```python
from build123d import *

# Parameters (mm, degrees)
ESQUISSE2_R             = 45
ESQUISSE2_R_2           = 1.55
BOSS_EXTRU_1_DEPTH      = 6.5
ENL_V_START             = -1.5
ESQUISSE3_R             = 45
ESQUISSE3_R_2           = 6
ENL_V_MAT_EXTRU_1_DEPTH = 1.5
CONG_1_R                = 0.1
ESQUISSE5_R             = 4
ENL_V_MAT_EXTRU_3_DEPTH = 5.5
SKETCH1_R               = 2.25
CUT_EXTRUDE1_DEPTH      = 64.835726815
SKETCH2_R               = 1.05
CUT_EXTRUDE2_DEPTH      = 64.970696557
CIRPATTERN1_COUNT       = 8
SKETCH6_R               = 6.9
CUT_EXTRUDE3_DEPTH      = 10
SKETCH7_R               = 5
CUT_EXTRUDE4_DEPTH      = 2.4


with BuildPart() as part:
    # Esquisse2 → Boss.-Extru.1 (new body)
    with BuildSketch(Plane(origin=(0, 0, 0), x_dir=(1, 0, 0), z_dir=(0, 1, 0))):
        with Locations(Location((0, 0, 0), (0, 0, 90))):
            Circle(ESQUISSE2_R)
        with Locations(Location((0, 0, 0), (0, 0, 90))):
            Circle(ESQUISSE2_R_2, mode=Mode.SUBTRACT)
    extrude(amount=BOSS_EXTRU_1_DEPTH)

    # Esquisse3 → Enlèv. mat.-Extru.1 (cut)
    with BuildSketch(Plane(origin=(0, 6.5, 0), x_dir=(1, 0, 0), z_dir=(0, 1, 0)).offset(ENL_V_START)):
        with Locations(Location((0, 0, 0), (0, 0, 90))):
            Circle(ESQUISSE3_R)
        with Locations(Location((0, 0, 0), (0, 0, 270))):
            Circle(ESQUISSE3_R_2, mode=Mode.SUBTRACT)
    extrude(amount=ENL_V_MAT_EXTRU_1_DEPTH, mode=Mode.SUBTRACT)

    # Congé1
    cong_1_edges = [part.edges().sort_by_distance(p)[0] for p in [
        (0, 5, 45),
        (0, 5, -6),
        (0, 6.5, -6),
        (0, 0, 45),
        (0, 6.5, 1.55),
    ]]
    fillet(cong_1_edges, radius=CONG_1_R)

    # Esquisse5 → Enlèv. mat.-Extru.3 (cut)
    with BuildSketch(Plane.XZ):
        with Locations(Location((0, 0, 0), (0, 0, 270))):
            Circle(ESQUISSE5_R)
    extrude(amount=-ENL_V_MAT_EXTRU_3_DEPTH, mode=Mode.SUBTRACT)

    # Sketch1 → Cut-Extrude1 (cut, through all)
    with BuildSketch(Plane(origin=(0, 5, 0), x_dir=(1, 0, 0), z_dir=(0, 1, 0))):
        with Locations(Location((0, 41.25, 0), (0, 0, 270))):
            Circle(SKETCH1_R)
        with Locations(Location((41.25, 0, 0), (0, 0, 270))):
            Circle(SKETCH1_R)
        with Locations(Location((0, -41.25, 0), (0, 0, 90))):
            Circle(SKETCH1_R)
        with Locations(Location((-41.25, 0, 0), (0, 0, 90))):
            Circle(SKETCH1_R)
    extrude(amount=-CUT_EXTRUDE1_DEPTH, mode=Mode.SUBTRACT)

    # Sketch2 → Cut-Extrude2 (cut, through all)
    with BuildSketch(Plane.XZ):
        with Locations(Location((0, 12, 0), (0, 0, 270))):
            Circle(SKETCH2_R)
    cut_extrude2 = extrude(amount=-CUT_EXTRUDE2_DEPTH, mode=Mode.SUBTRACT)

    # CirPattern1: Cut-Extrude2 ×8 about axis
    cirpattern1_axis = Axis((0, 0, 0), (0, 1, 0))
    for i in range(1, CIRPATTERN1_COUNT):
        add(cut_extrude2.rotate(cirpattern1_axis, i * 360 / CIRPATTERN1_COUNT), mode=Mode.SUBTRACT)

    # Sketch6 → Cut-Extrude3 (cut)
    with BuildSketch(Plane(origin=(0, 6.5, 0), x_dir=(1, 0, 0), z_dir=(0, 1, 0))):
        with Locations(Location((0, 0, 0), (0, 0, 270))):
            Circle(SKETCH6_R)
    extrude(amount=-CUT_EXTRUDE3_DEPTH, mode=Mode.SUBTRACT)

    # Sketch7 → Cut-Extrude4 (cut)
    with BuildSketch(Plane(origin=(0, 5, 0), x_dir=(1, 0, 0), z_dir=(0, 1, 0))):
        with Locations((-41.25, 0)):
            Circle(SKETCH7_R)
        with Locations((0, 41.25)):
            Circle(SKETCH7_R)
        with Locations((41.25, 0)):
            Circle(SKETCH7_R)
        with Locations((0, -41.25)):
            Circle(SKETCH7_R)
    extrude(amount=-CUT_EXTRUDE4_DEPTH, mode=Mode.SUBTRACT)


solid = part.part
```
Check sheet for the modelled part. Datum: model origin and axes. Units: mm. A direction names the side the tool comes from. Round coordinates to 2 decimals unless told otherwise and drop trailing zeros. Write item = value, one per line. Start each with the question number.
1) Sectioned sample at A-A, the plane x = 0. State how many separate pieces and enclosed holes the cut face has, plus the area to 3 significant figures.
2) Gauge pin test, flat ends, axial feed: pin 1 Ø6 at (x, z) = (0, 41.25) entering from -Y; pin 2 Ø3 at (x, y) = (22, 3) entering from +Z; pin 3 Ø3 at (x, y) = (31.5, 3) entering from -Z; pin 4 Ø3 at (x, y) = (35, 3.5) entering from +Z. Record the tip position at first contact, or that the pin passes through.
3) Set-up check for faces 3 (the cylindrical face through (-0.4, 2.46, 11.03)), 4 (the flat face through (-38.7, 2.6, -0.1)): record each of +Z, -Z, +X, -X, +Y, -Y from which the full face is reachable in a straight line by a thin tool's end or side.
4) Thickness scan on probe 1 along Z at (x, y) = (-9, 3.3); probe 2 along Z at (x, y) = (0.5, 3.2); probe 3 along Z at (x, y) = (12, 4.05). Record the ranges inside material, lowest first.
5) Release check for a two-part mould opening along X. For faces 1 (the flat face through (9, 0, 1)), 2 (the cylindrical face through (-11.03, 2.46, -0.4)) record: released by +X, released by -X, zero draft, split by the parting line, or undercut.
Results are:
q1.separate_pieces = 6
q1.enclosed_holes = 0
q1.area = 295 mm^2
q2.pin_1 = 0
q2.pin_2 = 40.06
q2.pin_3 = -33.54
q2.pin_4 = 30.05
q3.face_3 = +Y, -Y
q3.face_4 = +Y
q4.probe_1 = -44.09 to -9.4, -7.57 to 7.57, 9.4 to 44.09
q4.probe_2 = -36.28 to -12.92, -11.08 to -6.88, 6.88 to 11.08, 12.92 to 36.28
q4.probe_3 = -43.37 to -1.05, 1.05 to 43.37
q5.face_1 = zero draft
q5.face_2 = undercut
